```python
from build123d import *

# Parameters (mm, degrees)
SKETCH_1_R          = 2.75
EXTRUDE_1_DEPTH     = 8
CUT_EXTRUDE_1_DEPTH = 7
EXTRUDE_2_DEPTH     = 3.5
EXTRUDE_START       = -8
SKETCH_5_R          = 7.5
SKETCH_5_R_2        = 2.75
EXTRUDE_3_DEPTH     = 8
SWEEP_1_PROFILE_R   = 1
SKETCH_47_R         = 7.5
SKETCH_47_R_2       = 3.25
CUT_EXTRUDE_3_DEPTH = 1.5
SKETCH_48_R         = 0.8
CUT_EXTRUDE_4_DEPTH = 3.7
CUT_EXTRUDE_6_DEPTH = 3.5


with BuildPart() as part:
    # 草图1 → 凸台-拉伸1 (new body)
    with BuildSketch(Plane(origin=(0, 0, 0), x_dir=(1, 0, 0), z_dir=(0, 1, 0))):
        with Locations(Location((0, 0, 0), (0, 0, 270))):
            Circle(SKETCH_1_R)
    extrude(amount=EXTRUDE_1_DEPTH)

    # 草图2 → 切除-拉伸1 (cut)
    with BuildSketch(Plane(origin=(0, 8, 0), x_dir=(1, 0, 0), z_dir=(0, 1, 0))):
        with BuildLine():
            Line((1.843908891, 1.2), (-1.843908891, 1.2))
            ThreePointArc((-1.843908891, 1.2), (-2.2, 0), (-1.843908891, -1.2))
            Line((-1.843908891, -1.2), (1.843908891, -1.2))
            ThreePointArc((1.843908891, -1.2), (2.109099282, -0.625859584), (2.2, 0))
            ThreePointArc((2.2, 0), (2.109099282, 0.625859584), (1.843908891, 1.2))
        make_face()
    extrude(amount=-CUT_EXTRUDE_1_DEPTH, mode=Mode.SUBTRACT)

    # 草图4 → 凸台-拉伸2 (add)
    with BuildSketch(Plane(origin=(0, 8, 0), x_dir=(1, 0, 0), z_dir=(0, 1, 0))):
        with BuildLine():
            ThreePointArc((1.6, 1.2), (0, 2), (-1.6, 1.2))
            Line((-1.6, 1.2), (1.6, 1.2))
        make_face()
        with BuildLine():
            ThreePointArc((-1.6, -1.2), (0, -2), (1.6, -1.2))
            Line((1.6, -1.2), (-1.6, -1.2))
        make_face()
    extrude(amount=EXTRUDE_2_DEPTH)

    # 草图5 → 凸台-拉伸3 (add)
    with BuildSketch(Plane(origin=(0, 8, 0), x_dir=(1, 0, 0), z_dir=(0, 1, 0)).offset(EXTRUDE_START)):
        with Locations(Location((0, 0, 0), (0, 0, 270))):
            Circle(SKETCH_5_R)
        Circle(SKETCH_5_R_2, mode=Mode.SUBTRACT)
    extrude(amount=EXTRUDE_3_DEPTH)

    # 切除-扫描1: sweep along a path in 草图16
    with BuildLine(Plane(origin=(0, 4.5, 0), x_dir=(-1, 0, 0), z_dir=(0, -1, 0))) as sweep_1_path:
        CenterArc((0, 0), 6.8, 0, 360)
    # 切除-扫描1 profile (on start of the path) → 切除-扫描1 (sweep, cut)
    with BuildSketch(Plane(origin=(-6.8, 4.5, 0), x_dir=(-1, 0, 0), z_dir=(0, 0, -1))):
        Circle(SWEEP_1_PROFILE_R)
    sweep(path=sweep_1_path.line, mode=Mode.SUBTRACT)

    # 草图47 → 切除-拉伸3 (cut)
    with BuildSketch(Plane.XZ):
        with Locations(Location((0, 0, 0), (0, 0, 270))):
            Circle(SKETCH_47_R)
        with Locations(Location((0, 0, 0), (0, 0, 270))):
            Circle(SKETCH_47_R_2, mode=Mode.SUBTRACT)
    extrude(amount=-CUT_EXTRUDE_3_DEPTH, mode=Mode.SUBTRACT)

    # 草图48 → 切除-拉伸4 (cut)
    with BuildSketch(Plane.XZ.offset(-1.5)):
        with Locations(Location((-5.7, 0, 0), (0, 0, 270))):
            Circle(SKETCH_48_R)
    extrude(amount=-CUT_EXTRUDE_4_DEPTH, mode=Mode.SUBTRACT)

    # 草图56 → 切除-拉伸6 (cut)
    with BuildSketch(Plane(origin=(0, 8, 0), x_dir=(1, 0, 0), z_dir=(0, 1, 0))):
        with BuildLine():
            Line((1.6, -1.2), (-1.6, -1.2))
            ThreePointArc((-1.6, -1.2), (0, -2), (1.6, -1.2))
        make_face()
        with BuildLine():
            Line((-1.6, 1.2), (1.6, 1.2))
            ThreePointArc((1.6, 1.2), (0, 2), (-1.6, 1.2))
        make_face()
    extrude(amount=CUT_EXTRUDE_6_DEPTH, mode=Mode.SUBTRACT)


solid = part.part
```
CAD build for the part. Positions are in the model's coordinates, mm. A direction names the side the tool comes from. Give positions to 0.01 mm unless a question says otherwise; leave off trailing zeros. Loops run counter-clockwise (first coordinate to the right, second up) from the corner with the lowest first, then second, coordinate; pieces in that order, holes last. Notation, with made-up numbers: M -24,-4.75 L -18,-4.75 A17 ccw -18,5.25 Z; hole C 20.25,-36.75 d4. An arc over 180 degrees is marked long. Use one line per item in the form item = value.
Item 1: Slice it at C-C (y = 5). List the corners of the cut face in (x, z).
Determined:
outline = M -5.88,-0.78 A5.93 ccw long -5.88,0.78 A0.8 cw long Z; hole M -1.84,-1.2 L 1.84,-1.2 A2.2 ccw 1.84,1.2 L -1.84,1.2 A2.2 ccw Z
Item 2: Two-plate mould, pull along X, no slides. Class faces 1 (the face through (0, 8, 2)), 2 (the face through (0, 5, 1.2)), 3 (the face through (-1.978, 0.74, 2.579)): pulls with the +X half, pulls with the -X half, needs draft (parallel to the pull), parting line crosses it, or undercut.
Determined:
face_1 = needs draft
face_2 = undercut
face_3 = parting line crosses it
Item 3: Which spindle directions (+Z, -Z, +X, -X, +Y, -Y) get a long thin tool onto all of the face, cutting with end or side? Do faces 4 (the face through (0, 5, -1.2)), 5 (the face through (0.33, 6.588, -7.493)), 6 (the face through (-4.907, 2.913, 0.104)). Say none if no direction does.
Determined:
face_4 = +Y
face_5 = +Y, -Y
face_6 = -Y
Item 4: Slice it at A-A (x = 0). List the corners of the cut face in (y, z), plus the area to 3 significant figures.
Determined:
outline = M 0,-3.25 L 1.5,-3.25 L 1.5,-7.5 L 3.79,-7.5 A1 cw long 5.21,-7.5 L 8,-7.5 L 8,-1.2 L 1,-1.2 L 1,1.2 L 8,1.2 L 8,7.5 L 5.21,7.5 A1 cw long 3.79,7.5 L 1.5,7.5 L 1.5,3.25 L 0,3.25 Z
area = 84.8 mm2
Item 5: Flat gauge pins, fed straight in: pin 1 (2.5 mm diameter, centred on x = -5.7, z = 0, fed in from -Y); pin 2 (1.5 mm diameter, centred on x = -1.5, y = 2, fed in from +Z); pin 3 (1.9 mm diameter, centred on x = -0.5, z = 0, fed in from +Y). Where does each tip first touch, or does it go through?
Determined:
pin_1 = 1.5
pin_2 = 7.46
pin_3 = 1
Item 6: Drill centre lines: probe 1 along Y at (x, z) = (-1.5, 4.25); probe 2 along Z at (x, y) = (0, 1.75); probe 3 along Z at (x, y) = (-5.7, 2.6). Where is each one in solid material? Low to high. Write a range as from..to.
Determined:
probe_1 = 1.5..8
probe_2 = -7.5..-1.2, 1.2..7.5
probe_3 = -4.87..-0.8, 0.8..4.87
Item 7: Slice it at B-B (y = 7.25). List the corners of the cut face in (x, z), plus the area to 3 significant figures.
Determined:
outline = C 0,0 d15; hole M -1.84,-1.2 L 1.84,-1.2 A2.2 ccw 1.84,1.2 L -1.84,1.2 A2.2 ccw Z
area = 167 mm2
